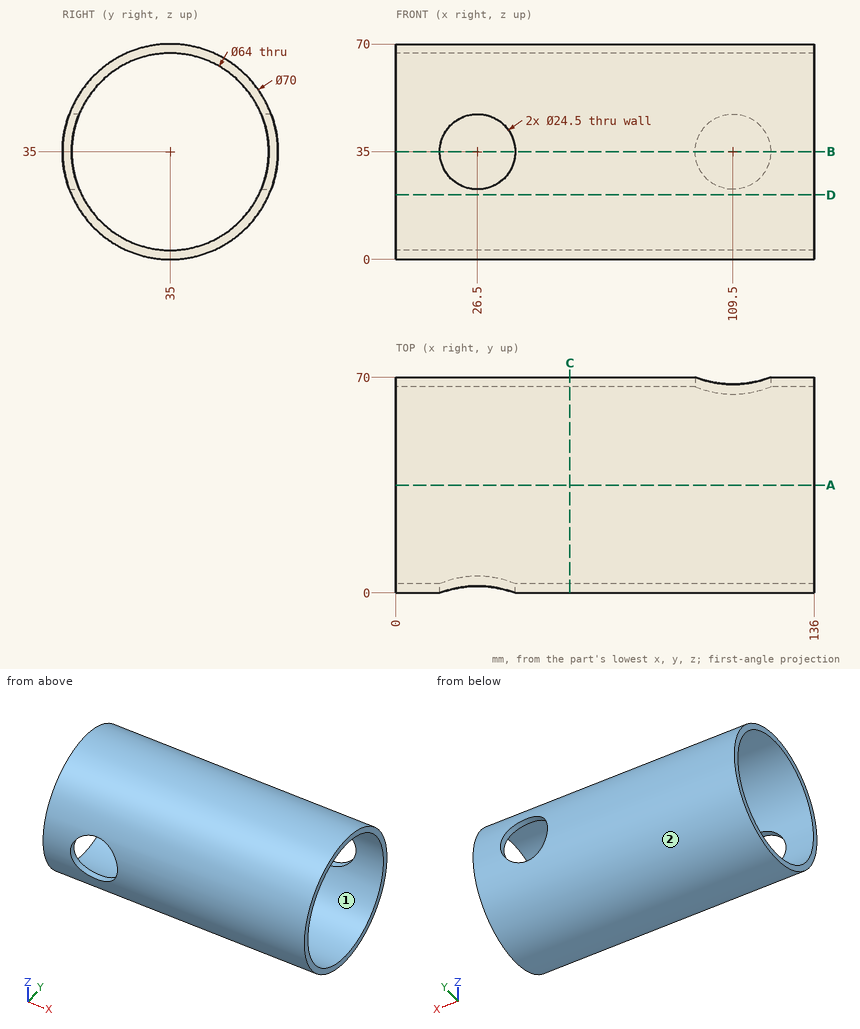
Can you work these out from the drawing? Everything is in mm from the part's minimum corner. Coordinates: 2 decimals unless noted, no trailing zeros. Write each loop counter-clockwise with the first axis right and the second up, starting at its lowest first coordinate (ties: lowest second). Pieces come first, ordered by that corner, then holes. Notation, with made-up numbers: (71, 33.25) -> (94, 33.25) arc R18 ccw to (94, 40.25) -> close; hole circle Ø1 at (-3, -28.5). An arc over 180 degrees is marked (long way). Return JSON: item names as keys, results as strings.
(1) Imagine slicing it at C-C, the plane x = 56.5. Please give me the cut outline in (y, z).
Numbers:
{"outline": "circle Ø70 at (35, 35); hole circle Ø64 at (35, 35)"}
(2) I'm going to push flat-ended pins straight in: pin 1 (8 mm diameter, centred on x = 94, y = 10.5, fed in from -Z); pin 2 (2 mm diameter, centred on x = 22, z = 45.5, fed in from +Y); pin 3 (19.5 mm diameter, centred on x = 109.5, z = 35, fed in from +Y). Where does each tip first touch, or does it pass through?
Numbers:
{"pin 1": "stops at z = 6.63", "pin 2": "stops at y = 68.69", "pin 3": "stops at y = 4.52"}
(3) I need wall thicknesses on L1, parallel to Y at x = 81.5, z = 35; L2, parallel to X at y = 1.6, z = 35; L3, parallel to X at y = 67.15, z = 35. Which ranges of each line are inside material? Lowest first, please.
Numbers:
{"L1": "y = 0 to 3, 67 to 70", "L2": "x = 0 to 14.25, 38.75 to 136", "L3": "x = 0 to 97.25, 121.75 to 136"}
(4) Imagine slicing it at B-B, the plane z = 35. Please give me the cut outline in (x, y).
Numbers:
{"outline": "(0, 0) -> (14.25, 0) -> (14.25, 3) -> (0, 3) -> close; (0, 67) -> (97.25, 67) -> (97.25, 70) -> (0, 70) -> close; (38.75, 0) -> (136, 0) -> (136, 3) -> (38.75, 3) -> close; (121.75, 67) -> (136, 67) -> (136, 70) -> (121.75, 70) -> close"}
(5) Imagine slicing it at D-D, the plane z = 21. Please give me the cut outline in (x, y).
Numbers:
{"outline": "(0, 2.92) -> (136, 2.92) -> (136, 6.23) -> (0, 6.23) -> close; (0, 63.77) -> (136, 63.77) -> (136, 67.08) -> (0, 67.08) -> close"}
(6) Imagine slicing it at A-A, the plane y = 35. Please give me the cut outline in (x, z).
Numbers:
{"outline": "(0, 0) -> (136, 0) -> (136, 3) -> (0, 3) -> close; (0, 67) -> (136, 67) -> (136, 70) -> (0, 70) -> close"}
(7) We'd pull the mould along Y, two halves only. Please class the marked faces 1 and 2: +Y half, -Y half, draft (parallel to the pull), parting line (faces both ways), or undercut.
Numbers:
{"face 1": "undercut", "face 2": "parting line"}
